Verification items for the finished model (mm, model axes). A direction names the side the tool comes from. Give positions to 0.01 mm unless a question says otherwise; leave off trailing zeros. Write each loop counter-clockwise with the first axis right and the second up, starting at its lowest first coordinate (ties: lowest second). Pieces come first, ordered by that corner, then holes. Notation, with made-up numbers: (-5.5, -16.5) -> (15.5, -16.5) arc R4 cw to (15.5, -10.5) -> close; hole circle Ø11 at (57.25, 76). An arc over 180 degrees is marked (long way). Use one line per item in the form item = value. Start each with the question number.
(1) Section check D-D, the plane y = -5.75. Record the cut outline in (x, z).
(2) Release check for a two-part mould opening along Z. For faces 1 (the face through (0, -6, -6.35)), 2 (the face through (0, -3, 3.175)), 3 (the face through (-6.35, -6, 0)) record: pulls with the +Z half, pulls with the -Z half, needs draft (parallel to the pull), parting line crosses it, or undercut.
(3) Section check A-A, the plane y = -2. Record the cut outline in (x, z) (3 decimals).
(4) Section check C-C, the plane x = -1.75. Record the cut outline in (y, z) (3 decimals).
(5) Section check B-B, the plane z = -1. Record the cut outline in (x, y) (3 decimals), plus the area to 3 significant figures.
(6) Set-up check for faces 4 (the face through (3.175, -3, 0)), 5 (the face through (3.33, -5.08, 0.05)), 6 (the face through (0, -6, 6.35)): record each of +Z, -Z, +X, -X, +Y, -Y from which the full face is reachable in a straight line by a thin tool's end or side.
(7) Scan lines: L1, parallel to Z at x = 0, y = -5 (3 decimals); L2, parallel to X at y = -6, z = 3.25; L3, parallel to Y at x = 3, z = 3. Record each from-to range of solid material in increasing order.
(8) Depth check by flat-ended pin: pin 1 Ø2.5 at (x, z) = (0.5, 0.5) entering from +Y. Enter the tip coordinate at first touch or a pass-through.
from build123d import *

# Parameters (mm, degrees)
F0_W     = 12.7
F0_H     = 12.7
F0_W_2   = 7.62
F0_H_2   = 7.62
F0_W_3   = 6.35
F0_H_3   = 6.35
F1_DEPTH = 12.7
F2_DEPTH = 7.62
F3_DEPTH = 7.62
F4_DEPTH = 5.08


with BuildPart() as f1:
    # F0 (on Front) → F1 (new body)
    with BuildSketch(Plane.XZ):
        Rectangle(F0_W, F0_H)
        Rectangle(F0_W_2, F0_H_2, mode=Mode.SUBTRACT)
        Rectangle(F0_W_2, F0_H_2)
        Rectangle(F0_W_3, F0_H_3, mode=Mode.SUBTRACT)
        Rectangle(F0_W_3, F0_H_3)
    extrude(amount=F1_DEPTH)

    # F0 (on Front) → F2 (cut)
    with BuildSketch(Plane.XZ):
        Rectangle(F0_W_3, F0_H_3)
    extrude(amount=F2_DEPTH, mode=Mode.SUBTRACT)

    # F0 (on Front) → F3 (cut)
    with BuildSketch(Plane.XZ):
        Rectangle(F0_W_2, F0_H_2)
        Rectangle(F0_W_3, F0_H_3, mode=Mode.SUBTRACT)
    extrude(amount=F3_DEPTH, mode=Mode.SUBTRACT)

    # F0 (on Front) → F4 (join)
    with BuildSketch(Plane.XZ):
        Rectangle(F0_W_2, F0_H_2)
        Rectangle(F0_W_3, F0_H_3, mode=Mode.SUBTRACT)
    extrude(amount=F4_DEPTH)


solid = f1.part
Completed:
q1.outline = (-6.35, -6.35) -> (6.35, -6.35) -> (6.35, 6.35) -> (-6.35, 6.35) -> close; hole (-3.81, -3.81) -> (3.81, -3.81) -> (3.81, 3.81) -> (-3.81, 3.81) -> close
q2.face_1 = pulls with the -Z half
q2.face_2 = undercut
q2.face_3 = needs draft
q3.outline = (-6.35, -6.35) -> (6.35, -6.35) -> (6.35, 6.35) -> (-6.35, 6.35) -> close; hole (-3.175, -3.175) -> (3.175, -3.175) -> (3.175, 3.175) -> (-3.175, 3.175) -> close
q4.outline = (-12.7, -6.35) -> (0, -6.35) -> (0, -3.175) -> (-5.08, -3.175) -> (-5.08, -3.81) -> (-7.62, -3.81) -> (-7.62, 3.81) -> (-5.08, 3.81) -> (-5.08, 3.175) -> (0, 3.175) -> (0, 6.35) -> (-12.7, 6.35) -> close
q5.outline = (-6.35, -12.7) -> (6.35, -12.7) -> (6.35, 0) -> (3.175, 0) -> (3.175, -5.08) -> (3.81, -5.08) -> (3.81, -7.62) -> (-3.81, -7.62) -> (-3.81, -5.08) -> (-3.175, -5.08) -> (-3.175, 0) -> (-6.35, 0) -> close
q5.area = 110 mm²
q6.face_4 = +Y
q6.face_5 = none
q6.face_6 = +Z, +X, -X, +Y, -Y
q7.L1 = -6.35 to -3.175, 3.175 to 6.35
q7.L2 = -6.35 to -3.81, 3.81 to 6.35
q7.L3 = -12.7 to -7.62
q8.pin_1 = -7.62
